```python
from build123d import *

# Parameters (mm, degrees)
PAD_DEPTH         = 50
SKETCH001_R       = 3.35
POCKET_DEPTH      = 130.001
POCKET_DEPTH_BACK = -4.001
SKETCH002_R       = 7
POCKET001_DEPTH   = 0.501
FILLET_R          = 10
FILLET001_R       = 2
SKETCH003_W       = 9
SKETCH003_H       = 12
POCKET002_DEPTH   = 29.001
SKETCH004_W       = 9
SKETCH004_H       = 12
POCKET003_DEPTH   = 4.001


with BuildPart() as part:
    # Sketch → Pad (new body)
    with BuildSketch(Plane.XY):
        Polygon((0, 130), (0, 0), (65, 0), (65, -4), (-29, -4), (-29, 0), (-4, 0), (-4, 126), (-9, 126), (-9, 120), (-13, 120), (-13, 130), align=None)
    extrude(amount=PAD_DEPTH)

    # Sketch001 → Pocket (cut, two sides)
    with BuildSketch(Plane.XZ) as pocket_sk:
        with Locations((45, 25)):
            Circle(SKETCH001_R)
    extrude(amount=-POCKET_DEPTH, mode=Mode.SUBTRACT)
    extrude(pocket_sk.sketch, amount=-POCKET_DEPTH_BACK, mode=Mode.SUBTRACT)

    # Sketch002 → Pocket001 (cut, through all)
    with BuildSketch(Plane.XZ.offset(3.5)):
        with Locations((45, 25)):
            Circle(SKETCH002_R)
    extrude(amount=POCKET001_DEPTH, mode=Mode.SUBTRACT)

    # Fillet
    fillet_edges = [part.edges().sort_by_distance(p)[0] for p in [
        (65, -2, 50),
        (65, -2, 0),
    ]]
    fillet(fillet_edges, radius=FILLET_R)

    # Fillet001
    fillet001_edges = [part.edges().sort_by_distance(p)[0] for p in [
        (-13, 130, 25),
        (0, 130, 25),
    ]]
    fillet(fillet001_edges, radius=FILLET001_R)

    # Sketch003 → Pocket002 (cut, through all)
    with BuildSketch(Plane.YZ):
        with Locations((4.5, 25)):
            Rectangle(SKETCH003_W, SKETCH003_H)
    extrude(amount=-POCKET002_DEPTH, mode=Mode.SUBTRACT)

    # Sketch004 → Pocket003 (cut, through all)
    with BuildSketch(Plane.XZ):
        with Locations((-24.5, 25)):
            Rectangle(SKETCH004_W, SKETCH004_H)
    extrude(amount=POCKET003_DEPTH, mode=Mode.SUBTRACT)


solid = part.part
```
CAD build for the part. Positions are in the model's coordinates, mm. A direction names the side the tool comes from. Give positions to 0.01 mm unless a question says otherwise; leave off trailing zeros. Loops run counter-clockwise (first coordinate to the right, second up) from the corner with the lowest first, then second, coordinate; pieces in that order, holes last. Notation, with made-up numbers: M 5,47.5 L 20,47.5 A9 ccw 20,51.5 Z; hole C 86.5,65.5 d3. An arc over 180 degrees is marked long. Use one line per item in the form item = value.
Item 1: Which spindle directions (+Z, -Z, +X, -X, +Y, -Y) get a long thin tool onto all of the face, cutting with end or side? Do faces 5 (the face through (-11, 120, 25)), 6 (the face through (-25, -2, 31)), 7 (the face through (0, 65, 25)). Say none if no direction does.
Determined:
face_5 = +Z, -Z, -X
face_6 = -X, +Y, -Y
face_7 = +Z, -Z, +X, +Y
Item 2: Slice it at A-A (x = -21.5). List the corners of the cut face in (y, z).
Determined:
outline = M -4,0 L 0,0 L 0,19 L -4,19 Z; M -4,31 L 0,31 L 0,50 L -4,50 Z
Item 3: Two-plate mould, pull along Z, no slides. Class faces 1 (the face through (-25, -2, 19)), 2 (the face through (-2, 38, 50)), 3 (the face through (-2, 4, 19)), 4 (the face through (-29, -2, 9)): pulls with the +Z half, pulls with the -Z half, needs draft (parallel to the pull), parting line crosses it, or undercut.
Determined:
face_1 = undercut
face_2 = pulls with the +Z half
face_3 = undercut
face_4 = needs draft
Item 4: Drill centre lines: probe 1 along X at (y, z) = (-0.7, 25); probe 2 along Z at (x, y) = (45, -2.5); probe 3 along Z at (x, y) = (45, -3.65). Where is each one in solid material? Low to high. Write a range as from..to.
Determined:
probe_1 = -20..41.65, 48.35..65
probe_2 = 0..21.65, 28.35..50
probe_3 = 0..18, 32..50
Item 5: Flat gauge pins, fed straight in: pin 1 (8 mm diameter, centred on x = 11.5, z = 40.5, fed in from +Y); pin 2 (5 mm diameter, centred on y = 122, z = 29.5, fed in from +X); pin 3 (1.2 mm diameter, centred on y = -3, z = 24.5, fed in from -X); pin 4 (15.5 mm diameter, centred on x = 45.5, z = 27, fed in from -Y). Where does each tip first touch, or does it go through?
Determined:
pin_1 = 0
pin_2 = 0
pin_3 = -20
pin_4 = -4
Item 6: Slice it at C-C (x = 45). List the corners of the cut face in (y, z), plus the area to 3 significant figures.
Determined:
outline = M -4,0 L 0,0 L 0,21.65 L -3.5,21.65 L -3.5,18 L -4,18 Z; M -4,32 L -3.5,32 L -3.5,28.35 L 0,28.35 L 0,50 L -4,50 Z
area = 170 mm2
Item 7: Slice it at B-B (z = 25). List the corners of the cut face in (x, y), plus the area to 3 significant figures.
Determined:
outline = M -20,-4 L 38,-4 L 38,-3.5 L 41.65,-3.5 L 41.65,0 L -20,0 Z; M -13,120 L -9,120 L -9,126 L -4,126 L -4,9 L 0,9 L 0,128 A2 ccw -2,130 L -11,130 A2 ccw -13,128 Z; M 48.35,-3.5 L 52,-3.5 L 52,-4 L 65,-4 L 65,0 L 48.35,0 Z
area = 852 mm2
Item 8: Slice it at D-D (y = 21.5). List the corners of the cut face in (x, z), plus the area to 3 significant figures.
Determined:
outline = M -4,0 L 0,0 L 0,50 L -4,50 Z
area = 200 mm2
